from build123d import *

# Parameters (mm, degrees)
SKETCH2_R          = 3.2639
CUT_EXTRUDE1_DEPTH = 79.267453006
CIRPATTERN1_COUNT  = 12


with BuildPart() as part:
    # Sketch1 → Revolve1 (revolve)
    with BuildSketch(Plane.XY, mode=Mode.PRIVATE) as revolve1_sk:
        Polygon((-9.525, 54.61), (9.525, 54.61), (9.525, 49.53), (3.175, 49.53), (3.175, 24.13), (5.715, 24.13), (5.715, 20.32), (-5.715, 20.32), (-5.715, 24.13), (-3.175, 24.13), (-3.175, 49.53), (-9.525, 49.53), align=None)
    revolve(revolve1_sk.sketch.rotate(Axis((-31.293370787, 0, 0), (1, 0, 0)), 90), axis=Axis((-31.293370787, 0, 0), (1, 0, 0)))

    # Sketch2 → Cut-Extrude1 (cut, through all)
    with BuildSketch(Plane(origin=(3.175, 0, 0), x_dir=(0, 0, -1), z_dir=(1, 0, 0))):
        with Locations((0, 30.48)):
            Circle(SKETCH2_R)
    cut_extrude1 = extrude(amount=-CUT_EXTRUDE1_DEPTH, mode=Mode.SUBTRACT)

    # CirPattern1: Cut-Extrude1 ×12 about axis
    cirpattern1_axis = Axis((0, 0, 0), (1, 0, 0))
    for i in range(1, CIRPATTERN1_COUNT):
        add(cut_extrude1.rotate(cirpattern1_axis, i * 360 / CIRPATTERN1_COUNT), mode=Mode.SUBTRACT)


solid = part.part
Source: CAD feature listing. Evaluate the final solid. Frame: model axes, mm. A direction names the side the tool comes from. Round coordinates to 2 decimals unless told otherwise and drop trailing zeros. Order: outer loops, then holes, each group sorted by start corner. A loop starts at its lowest first (then second) coordinate and runs counter-clockwise, first axis right, second up. Notation, with made-up numbers: (-26.5, -34.75) - (7.5, -34.75) arc R8 ccw to (7.5, -28.75) - close; hole circle Ø2 at (86.5, 60). An arc over 180 degrees is marked (long way). Use a Markdown table: item, result. Add a question column.
1. Set-up query: faces 1 (the cylindrical face through (6.31, -14.88, 47.24)), 2 (the flat face through (-5.715, 16, 13)), 3 (the cylindrical face through (0.044, -18.136, 24.89)). Return all of +Z, -Z, +X, -X, +Y, -Y with unobstructed straight access to the full face (end or side cutting, diameter ignored); none if empty.
2. Mould query, pull axis Y, two halves, no side actions, for faces 4 (the cylindrical face through (0.044, -24.89, -18.136)), 5 (the cylindrical face through (0.133, -54.145, -7.109)), 6 (the flat face through (-9.525, 48.3, -11.9)). Classes: +Y half, -Y half, draft (parallel to the pull), parting line (faces both ways), or undercut.
3. Section query D-D (y = -46). Return the cut outline in (x, z) (3 decimals), then the cut area to 3 significant figures.
4. Section query A-A (y = 0). Give the number of separate pieces and of enclosed holes in the cut face, then the cut area to 3 significant figures.
5. First-contact query: pin 1 (8 mm diameter, centred on x = 4.5, z = 29, fed in from +Y); pin 2 (1.5 mm diameter, centred on x = 5, z = -41.5, fed in from -Y); pin 3 (7.5 mm diameter, centred on y = 15.24, z = -26.4, fed in from -X) (3 decimals); pin 4 (12 mm diameter, centred on y = 36, z = -30.5, fed in from +X) (3 decimals). Flat tips, straight axial feed; report the tip coordinate or a pass-through.
6. Line query: probe 1 along Y at (x, z) = (-0.25, 0); probe 2 along Y at (x, z) = (-3.5, 1.5); probe 3 along Z at (x, y) = (-0.75, -15.5). Output: solid intervals per line, ascending.
Derived:
| question | item | result |
|---|---|---|
| 1 | face 1 | +X |
| 1 | face 2 | -X |
| 1 | face 3 | +X, -X |
| 2 | face 4 | undercut |
| 2 | face 5 | parting line |
| 2 | face 6 | draft |
| 3 | outline | (-9.525, -29.432) - (9.525, -29.432) - (9.525, -18.364) - (3.175, -18.364) - (3.175, 18.364) - (9.525, 18.364) - (9.525, 29.432) - (-9.525, 29.432) - (-9.525, 18.364) - (-3.175, 18.364) - (-3.175, -18.364) - (-9.525, -18.364) - close |
| 3 | area | 655 mm2 |
| 4 | separate pieces | 4 |
| 4 | enclosed holes | 0 |
| 4 | area | 520 mm2 |
| 5 | pin 1 | y = 48.55 |
| 5 | pin 2 | y = -36.36 |
| 5 | pin 3 | x = -3.175 |
| 5 | pin 4 | x = 9.525 |
| 6 | probe 1 | -54.61 to -33.74, -27.22 to -20.32, 20.32 to 27.22, 33.74 to 54.61 |
| 6 | probe 2 | -54.59 to -49.51, -24.08 to -20.26, 20.26 to 24.08, 49.51 to 54.59 |
| 6 | probe 3 | -52.36 to -29.65, -23.14 to -13.14, 13.14 to 23.14, 29.65 to 52.36 |
